```python
from build123d import *

# Parameters (mm, degrees)
F1_W      = 50
F1_H      = 120
F2_DEPTH  = 25
F3_W      = 40
F3_H      = 40
F4_DEPTH  = 50
F5_W      = 25
F5_H      = 40
F6_DEPTH  = 50
F7_W      = 25
F7_H      = 40
F8_DEPTH  = 50
F9_W      = 30
F9_H      = 10
F10_DEPTH = 50
F11_W     = 30
F11_H     = 10
F12_DEPTH = 70
F13_W     = 30
F13_H     = 10
F14_DEPTH = 70


with BuildPart() as f2:
    # F1 (on Top) → F2 (new body, symmetric)
    with BuildSketch(Plane.XY):
        Rectangle(F1_W, F1_H)
    extrude(amount=F2_DEPTH, both=True)

    # F3 (on face) → F4 (cut)
    with BuildSketch(Plane(origin=(-25, 0, 0), x_dir=(0, -1, 0), z_dir=(-1, 0, 0))):
        with Locations((0, -25)):
            Rectangle(F3_W, F3_H)
    extrude(amount=-F4_DEPTH, mode=Mode.SUBTRACT)

    # F5 (on face) → F6 (cut)
    with BuildSketch(Plane(origin=(-25, 0, 0), x_dir=(0, -1, 0), z_dir=(-1, 0, 0))):
        with Locations((-47.5, 5)):
            Rectangle(F5_W, F5_H)
    extrude(amount=-F6_DEPTH, mode=Mode.SUBTRACT)

    # F7 (on face) → F8 (cut)
    with BuildSketch(Plane(origin=(-25, 0, 0), x_dir=(0, -1, 0), z_dir=(-1, 0, 0))):
        with Locations((47.5, 5)):
            Rectangle(F7_W, F7_H)
    extrude(amount=-F8_DEPTH, mode=Mode.SUBTRACT)

    # F9 (on face) → F10 (cut)
    with BuildSketch(Plane(origin=(-25, 0, 0), x_dir=(0, -1, 0), z_dir=(-1, 0, 0))):
        with Locations((0, 20)):
            Rectangle(F9_W, F9_H)
    extrude(amount=-F10_DEPTH, mode=Mode.SUBTRACT)

    # F11 (on face) → F12 (cut)
    with BuildSketch(Plane.XZ.offset(35)):
        with Locations((0, 20)):
            Rectangle(F11_W, F11_H)
    extrude(amount=-F12_DEPTH, mode=Mode.SUBTRACT)

    # F13 (on face) → F14 (cut)
    with BuildSketch(Plane.XZ.offset(35)):
        with Locations((-0.1553255133, 10.0446071414)):
            Rectangle(F13_W, F13_H)
    extrude(amount=-F14_DEPTH, mode=Mode.SUBTRACT)


solid = f2.part
```
The listing builds one solid part. Answer for the finished solid, in the listing's coordinates (mm). A direction names the side the tool comes from. Give positions to 0.01 mm unless a question says otherwise; leave off trailing zeros. Loops run counter-clockwise (first coordinate to the right, second up) from the corner with the lowest first, then second, coordinate; pieces in that order, holes last. Notation, with made-up numbers: (46.5, -32) - (65.5, -32) arc R8 cw to (65.5, -23) - close; hole circle Ø6 at (-13.5, 2.25). An arc over 180 degrees is marked (long way). Return JSON: item names as keys, results as strings. Group by question number.
1. Find section A-A (z = 20). Write down the section's boundary in (x, y).
2. Straight lines are drawn through the part: line 1 (Y direction, x = 8.5, z = -17); line 2 (X direction, y = -19.5, z = 10.5); line 3 (X direction, y = -17, z = 18). For each, find the intervals that lie inside material, in ascending order. Write a range as [from, to].
3. Find section B-B (z = 13). Write down the section's boundary in (x, y).
4. Which of the six approach directions +Z, -Z, +X, -X, +Y, -Y give full straight-line access (tool end or side, diameter ignored) to faces 4 (the flat face through (0, -20, -15)), 5 (the flat face through (20, 15, 20)), 6 (the flat face through (-20, 25, 25)), 7 (the flat face through (15, -25, 20)), 8 (the flat face through (0, -40, -25))?
5. Given pin 1 Ø3 at (x, z) = (20, 17.5) entering from -Y; pin 2 Ø8 at (x, y) = (-18.5, 3) entering from +Z; pin 3 Ø12 at (x, z) = (9, 2) entering from +Y, each flat-ended and moving along its own axis, determine where each tip first touches the part or whether it passes through.
6. Determine the mould class of faces 1 (the flat face through (-20, 0, 15)), 2 (the flat face through (-15, -25, 20)), 3 (the flat face through (-25, -1, 0)) for opening direction X: pulls with the +X half, pulls with the -X half, needs draft (parallel to the pull), parting line crosses it, or undercut.
7. Find section D-D (x = -19). Write down the section's boundary in (y, z), then the cut area to 3 significant figures.
8. Find section C-C (y = 18.5). Write down the section's boundary in (x, z).
Verdict:
{
 "1": {"outline": "(-25, -35) - (-15, -35) - (-15, -15) - (-25, -15) - close; (-25, 15) - (-15, 15) - (-15, 35) - (-25, 35) - close; (15, -35) - (25, -35) - (25, -15) - (15, -15) - close; (15, 15) - (25, 15) - (25, 35) - (15, 35) - close"},
 "2": {"line 1": "y = [-60, -20], [20, 60]", "line 2": "x = [-25, -15.16], [14.84, 25]", "line 3": "x = [-25, -15], [15, 25]"},
 "3": {"outline": "(-25, -35) - (-15.16, -35) - (-15.16, 35) - (-25, 35) - close; (14.84, -35) - (25, -35) - (25, 35) - (14.84, 35) - close"},
 "4": {"face 4": "-Z, +X, -X", "face 5": "+Z, +X, -X", "face 6": "+Z, +X, -X, +Y, -Y", "face 7": "+Z, +Y, -Y", "face 8": "-Z, +X, -X, +Y, -Y"},
 "5": {"pin 1": "stops at y = -35", "pin 2": "stops at z = 15", "pin 3": "stops at y = 35"},
 "6": {"face 1": "needs draft", "face 2": "undercut", "face 3": "pulls with the -X half"},
 "7": {"outline": "(-60, -25) - (-20, -25) - (-20, -5) - (20, -5) - (20, -25) - (60, -25) - (60, -15) - (35, -15) - (35, 25) - (15, 25) - (15, 15) - (-15, 15) - (-15, 25) - (-35, 25) - (-35, -15) - (-60, -15) - close", "area": "2,900 mm^2"},
 "8": {"outline": "(-25, -5) - (25, -5) - (25, 25) - (15, 25) - (15, 15) - (14.84, 15) - (14.84, 5.04) - (-15.16, 5.04) - (-15.16, 15.04) - (-15, 15.04) - (-15, 25) - (-25, 25) - close"}
}
